CAD build for the part. Positions are in the model's coordinates, mm. A direction names the side the tool comes from. Round coordinates to 2 decimals unless told otherwise and drop trailing zeros. Loops run counter-clockwise (first coordinate to the right, second up) from the corner with the lowest first, then second, coordinate; pieces in that order, holes last. Notation, with made-up numbers: M -5,-15 L 30,-15 A19 cw 30,16 Z; hole C 2,79 d6. An arc over 180 degrees is marked long. Use a Markdown table: item, result. Add a question column.
(1) Which spindle directions (+Z, -Z, +X, -X, +Y, -Y) get a long thin tool onto all of the face, cutting with end or side? Do faces 4 (the face through (-86.16, -52.426, 3.479)), 5 (the face through (-73, -26, 2)), 6 (the face through (96.168, 62.216, 0.986)). Say none if no direction does.
(2) Band-saw the part on C-C, the plane y = 45. Write the cut outline in (x, z), and give its area (3 significant figures).
(3) Band-saw the part on A-A, the plane x = 76. Write the cut outline in (y, z) (1 decimal).
(4) Flat gauge pins, fed straight in: P1, Ø0.9, axis at y = -17, z = 4, coming from the +X side; P2, Ø1.6, axis at y = -60.5, z = 1.5, coming from the +X side; P3, Ø0.9, axis at x = -73.5, z = 3.5, coming from the -Y side (3 decimals). Where does each tip first touch, or does it go through?
(5) Two-plate mould, pull along Y, no slides. Class faces 1 (the face through (45, -33, 2)), 2 (the face through (86.081, -52.505, 3.479)), 3 (the face through (-95.871, 62.513, 0.986)): released by +Y, released by -Y, zero draft, split by the parting line, or undercut.
(6) Wall check: L1, parallel to Y at x = 76, z = 1.5 (1 decimal); L2, parallel to Y at x = -68.5, z = 4.4 (3 decimals); L3, parallel to Y at x = -11, z = 2.4 (3 decimals). Give the ranges that are in metal, low to high.
(7) Band-saw the part on D-D, the plane x = -74. Write the cut outline in (y, z) (3 decimals), and give its area (3 significant figures).
from build123d import *

# Parameters (mm, degrees)
F0_R     = 2
F0_W     = 11.2
F0_H     = 30.8
F0_R_2   = 3.175
F1_DEPTH = 2
F2_W     = 72.0786
F2_H     = 54.5526
F2_R     = 1.651
F3_DEPTH = 2.001
F4_SIZE  = 1
F5_W     = 82.0786
F5_H     = 79.5526
F6_DEPTH = 3


with BuildPart() as f1:
    # F0 (on Top) → F1 (new body)
    with BuildSketch(Plane.XY):
        with BuildLine():
            Line((-82.55, -67.945), (82.55, -67.945))
            ThreePointArc((82.55, -67.945), (96.020384, -62.365384), (101.6, -48.895))
            Line((101.6, -48.895), (101.6, 48.895))
            ThreePointArc((101.6, 48.895), (96.020384, 62.365384), (82.55, 67.945))
            Line((82.55, 67.945), (-82.55, 67.945))
            ThreePointArc((-82.55, 67.945), (-96.020384, 62.365384), (-101.6, 48.895))
            Line((-101.6, 48.895), (-101.6, -48.895))
            ThreePointArc((-101.6, -48.895), (-96.020384, -62.365384), (-82.55, -67.945))
        make_face()
        with BuildLine():
            Line((-84.46, -59.585), (-84.46, -62.335))
            ThreePointArc((-84.46, -62.335), (-86.36, -64.235), (-88.26, -62.335))
            Line((-88.26, -62.335), (-88.26, -59.585))
            ThreePointArc((-88.26, -59.585), (-86.36, -57.685), (-84.46, -59.585))
        make_face(mode=Mode.SUBTRACT)
        with BuildLine():
            Line((1.9, -59.585), (1.9, -62.335))
            ThreePointArc((1.9, -62.335), (0, -64.235), (-1.9, -62.335))
            Line((-1.9, -62.335), (-1.9, -59.585))
            ThreePointArc((-1.9, -59.585), (0, -57.685), (1.9, -59.585))
        make_face(mode=Mode.SUBTRACT)
        with Locations((-94, -13.3)):
            Circle(F0_R, mode=Mode.SUBTRACT)
        with BuildLine():
            Line((88.26, -59.585), (88.26, -62.335))
            ThreePointArc((88.26, -62.335), (86.36, -64.235), (84.46, -62.335))
            Line((84.46, -62.335), (84.46, -59.585))
            ThreePointArc((84.46, -59.585), (86.36, -57.685), (88.26, -59.585))
        make_face(mode=Mode.SUBTRACT)
        with Locations((76, -6.5875)):
            Rectangle(F0_W, F0_H, mode=Mode.SUBTRACT)
        with Locations((94, -13.3)):
            Circle(F0_R, mode=Mode.SUBTRACT)
        with Locations((-94, 26.9)):
            Circle(F0_R, mode=Mode.SUBTRACT)
        with BuildLine():
            Line((-84.46, 62.335), (-84.46, 59.585))
            ThreePointArc((-84.46, 59.585), (-86.36, 57.685), (-88.26, 59.585))
            Line((-88.26, 59.585), (-88.26, 62.335))
            ThreePointArc((-88.26, 62.335), (-86.36, 64.235), (-84.46, 62.335))
        make_face(mode=Mode.SUBTRACT)
        with BuildLine():
            Line((1.9, 62.335), (1.9, 59.585))
            ThreePointArc((1.9, 59.585), (0, 57.685), (-1.9, 59.585))
            Line((-1.9, 59.585), (-1.9, 62.335))
            ThreePointArc((-1.9, 62.335), (0, 64.235), (1.9, 62.335))
        make_face(mode=Mode.SUBTRACT)
        with Locations((76, 18.8125)):
            Circle(F0_R_2, mode=Mode.SUBTRACT)
        with Locations((94, 26.9)):
            Circle(F0_R, mode=Mode.SUBTRACT)
        with BuildLine():
            Line((88.26, 62.335), (88.26, 59.585))
            ThreePointArc((88.26, 59.585), (86.36, 57.685), (84.46, 59.585))
            Line((84.46, 59.585), (84.46, 62.335))
            ThreePointArc((84.46, 62.335), (86.36, 64.235), (88.26, 62.335))
        make_face(mode=Mode.SUBTRACT)
    extrude(amount=F1_DEPTH)

    # F2 (on face) → F3 (cut, through all)
    with BuildSketch(Plane.XY.offset(2)):
        Rectangle(F2_W, F2_H)
        with Locations((-29.5656, 31.4579)):
            Circle(F2_R)
        with Locations((29.5656, 31.4579)):
            Circle(F2_R)
        with Locations((29.5656, -36.6141)):
            Circle(F2_R)
        with Locations((-29.5656, -36.6141)):
            Circle(F2_R)
    extrude(amount=-F3_DEPTH, mode=Mode.SUBTRACT)

    # F4
    f4_edges = [f1.edges().sort_by_distance(p)[0] for p in [
        (0, 27.2763, 0),
        (36.0393, 0, 0),
        (-36.0393, 0, 0),
        (0, -27.2763, 0),
    ]]
    chamfer(f4_edges, length=F4_SIZE)

    # F5 (on face) → F6 (join)
    with BuildSketch(Plane.XY.offset(2)):
        with BuildLine():
            Line((87.6, -48.895), (87.6, 48.895))
            ThreePointArc((87.6, 48.895), (86.120889, 52.465889), (82.55, 53.945))
            Line((82.55, 53.945), (-82.55, 53.945))
            ThreePointArc((-82.55, 53.945), (-86.120889, 52.465889), (-87.6, 48.895))
            Line((-87.6, 48.895), (-87.6, -48.895))
            ThreePointArc((-87.6, -48.895), (-86.120889, -52.465889), (-82.55, -53.945))
            Line((-82.55, -53.945), (82.55, -53.945))
            ThreePointArc((82.55, -53.945), (86.120889, -52.465889), (87.6, -48.895))
        make_face()
        with BuildLine():
            ThreePointArc((-82.55, -50.945), (-83.999569, -50.344569), (-84.6, -48.895))
            Line((-84.6, -48.895), (-84.6, -1.5))
            Line((-84.6, -1.5), (-61.81965, -1.5))
            Line((-61.81965, -1.5), (-61.81965, -50.945))
            Line((-61.81965, -50.945), (-82.55, -50.945))
        make_face(mode=Mode.SUBTRACT)
        Polygon((-44.0393, -1.5), (-44.0393, -45.2763), (-1.5, -45.2763), (-1.5, -50.945), (-58.81965, -50.945), (-58.81965, -1.5), align=None, mode=Mode.SUBTRACT)
        Polygon((58.81965, -1.5), (58.81965, -50.945), (1.5, -50.945), (1.5, -45.2763), (44.0393, -45.2763), (44.0393, -1.5), align=None, mode=Mode.SUBTRACT)
        with Locations((0, -2.5)):
            Rectangle(F5_W, F5_H, mode=Mode.SUBTRACT)
        with BuildLine():
            ThreePointArc((-84.6, 48.895), (-83.999569, 50.344569), (-82.55, 50.945))
            Line((-82.55, 50.945), (-61.81965, 50.945))
            Line((-61.81965, 50.945), (-61.81965, 1.5))
            Line((-61.81965, 1.5), (-84.6, 1.5))
            Line((-84.6, 1.5), (-84.6, 48.895))
        make_face(mode=Mode.SUBTRACT)
        Polygon((-58.81965, 1.5), (-58.81965, 50.945), (-1.5, 50.945), (-1.5, 40.2763), (-44.0393, 40.2763), (-44.0393, 1.5), align=None, mode=Mode.SUBTRACT)
        Polygon((1.5, 50.945), (58.81965, 50.945), (58.81965, 1.5), (44.0393, 1.5), (44.0393, 40.2763), (1.5, 40.2763), align=None, mode=Mode.SUBTRACT)
        with BuildLine():
            ThreePointArc((82.55, 50.945), (83.999569, 50.344569), (84.6, 48.895))
            Line((84.6, 48.895), (84.6, -48.895))
            ThreePointArc((84.6, -48.895), (83.999569, -50.344569), (82.55, -50.945))
            Line((82.55, -50.945), (61.81965, -50.945))
            Line((61.81965, -50.945), (61.81965, 50.945))
            Line((61.81965, 50.945), (82.55, 50.945))
        make_face(mode=Mode.SUBTRACT)
    extrude(amount=F6_DEPTH)


solid = f1.part
Return value:
| question | item | result |
|---|---|---|
| 1 | face 4 | +Z, -X, -Y |
| 1 | face 5 | +Z |
| 1 | face 6 | +Z, -Z, +X, +Y |
| 2 | outline | M -101.6,0 L 101.6,0 L 101.6,2 L 87.6,2 L 87.6,5 L 84.6,5 L 84.6,2 L 61.82,2 L 61.82,5 L 58.82,5 L 58.82,2 L 1.5,2 L 1.5,5 L -1.5,5 L -1.5,2 L -58.82,2 L -58.82,5 L -61.82,5 L -61.82,2 L -84.6,2 L -84.6,5 L -87.6,5 L -87.6,2 L -101.6,2 Z |
| 2 | area | 451 mm^2 |
| 3 | outline | M -67.9,0 L -22,0 L -22,2 L -50.9,2 L -50.9,5 L -53.9,5 L -53.9,2 L -67.9,2 Z; M 8.8,0 L 15.6,0 L 15.6,2 L 8.8,2 Z; M 22,0 L 67.9,0 L 67.9,2 L 53.9,2 L 53.9,5 L 50.9,5 L 50.9,2 L 22,2 Z |
| 4 | P1 | x = 87.6 |
| 4 | P2 | x = 98.24 |
| 4 | P3 | y = -53.945 |
| 5 | face 1 | undercut |
| 5 | face 2 | released by -Y |
| 5 | face 3 | released by +Y |
| 6 | L1 | -67.9 to -22, 8.8 to 15.6, 22 to 67.9 |
| 6 | L2 | -53.945 to -50.945, -1.5 to 1.5, 50.945 to 53.945 |
| 6 | L3 | -53.945 to -50.945, -45.276 to -42.276, 37.276 to 40.276, 50.945 to 53.945 |
| 7 | outline | M -67.945,0 L 67.945,0 L 67.945,2 L 53.945,2 L 53.945,5 L 50.945,5 L 50.945,2 L 1.5,2 L 1.5,5 L -1.5,5 L -1.5,2 L -50.945,2 L -50.945,5 L -53.945,5 L -53.945,2 L -67.945,2 Z |
| 7 | area | 299 mm^2 |
